from build123d import *

# Parameters (mm, degrees)
SKETCH_1_W          = 15
SKETCH_1_H          = 15
SKETCH_1_W_2        = 12
SKETCH_1_H_2        = 12
EXTRUDE_1_DEPTH     = 135
SKETCH_2_R          = 2.7
CUT_EXTRUDE_1_DEPTH = 25
SKETCH_3_R          = 2.7
SKETCH_3_R_2        = 2.25
CUT_EXTRUDE_2_DEPTH = 25
SKETCH_4_R          = 5
CUT_EXTRUDE_3_DEPTH = 10
SKETCH_5_R          = 5
CUT_EXTRUDE_4_DEPTH = 10
SKETCH_6_R          = 5
CUT_EXTRUDE_5_DEPTH = 10


with BuildPart() as part:
    # ｽｹｯﾁ1 → ﾎﾞｽ - 押し出し1 (new body)
    with BuildSketch(Plane.XY):
        Rectangle(SKETCH_1_W, SKETCH_1_H)
        Rectangle(SKETCH_1_W_2, SKETCH_1_H_2, mode=Mode.SUBTRACT)
    extrude(amount=EXTRUDE_1_DEPTH)

    # ｽｹｯﾁ2 → ｶｯﾄ - 押し出し1 (cut)
    with BuildSketch(Plane(origin=(7.5, 0, 0), x_dir=(0, 0, -1), z_dir=(1, 0, 0))):
        with Locations((-112.5, 0)):
            Circle(SKETCH_2_R)
        with Locations((-22.5, 0)):
            Circle(SKETCH_2_R)
    extrude(amount=-CUT_EXTRUDE_1_DEPTH, mode=Mode.SUBTRACT)

    # ｽｹｯﾁ3 → ｶｯﾄ - 押し出し2 (cut)
    with BuildSketch(Plane(origin=(0, 7.5, 0), x_dir=(1, 0, 0), z_dir=(0, 1, 0))):
        with Locations((0, -7.5)):
            Circle(SKETCH_3_R)
        with Locations((0, -127.5)):
            Circle(SKETCH_3_R_2)
    extrude(amount=-CUT_EXTRUDE_2_DEPTH, mode=Mode.SUBTRACT)

    # ｽｹｯﾁ4 → ｶｯﾄ - 押し出し3 (cut)
    with BuildSketch(Plane(origin=(0, 7.5, 0), x_dir=(1, 0, 0), z_dir=(0, 1, 0))):
        with Locations((0, -7.5)):
            Circle(SKETCH_4_R)
    extrude(amount=-CUT_EXTRUDE_3_DEPTH, mode=Mode.SUBTRACT)

    # ｽｹｯﾁ5 → ｶｯﾄ - 押し出し4 (cut)
    with BuildSketch(Plane(origin=(7.5, 0, 0), x_dir=(0, 0, -1), z_dir=(1, 0, 0))):
        with Locations((-22.5, 0)):
            Circle(SKETCH_5_R)
        with Locations((-112.5, 0)):
            Circle(SKETCH_5_R)
    extrude(amount=-CUT_EXTRUDE_4_DEPTH, mode=Mode.SUBTRACT)

    # ｽｹｯﾁ6 → ｶｯﾄ - 押し出し5 (cut)
    with BuildSketch(Plane(origin=(0, -7.5, 0), x_dir=(-1, 0, 0), z_dir=(0, -1, 0))):
        with Locations((0, -127.5)):
            Circle(SKETCH_6_R)
    extrude(amount=-CUT_EXTRUDE_5_DEPTH, mode=Mode.SUBTRACT)


solid = part.part
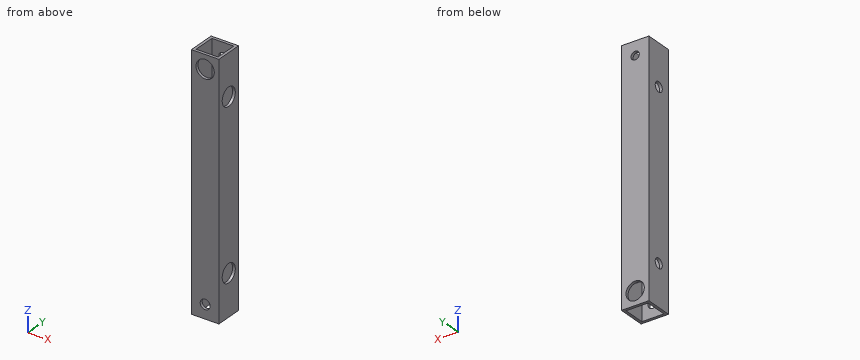
Verification items for the finished model (mm, model axes). Round coordinates to 2 decimals unless told otherwise and drop trailing zeros. Order: outer loops, then holes, each group sorted by start corner. A loop starts at its lowest first (then second) coordinate and runs counter-clockwise, first axis right, second up. Notation, with made-up numbers: (85.5, 10) -> (141.5, 10) arc R15 ccw to (141.5, 32) -> close; hole circle Ø2 at (-1, 70.25). An arc over 180 degrees is marked (long way). Put each result on its own line as item: value.
1) Depth check by flat-ended pin: pin 1 (5 mm diameter, centred on x = 0, z = 127.5, fed in from -Y); pin 2 (8 mm diameter, centred on x = 0, z = 7.5, fed in from -Y). Enter the tip coordinate at first touch or a pass-through.
Final values:
pin 1: stops at y = 6
pin 2: stops at y = -7.5
2) Section check D-D (z = 100). Record the cut outline in (x, y), then the cut area to 3 significant figures.
Final values:
outline: (-7.5, -7.5) -> (7.5, -7.5) -> (7.5, 7.5) -> (-7.5, 7.5) -> close; hole (-6, -6) -> (6, -6) -> (6, 6) -> (-6, 6) -> close
area: 81.0 mm^2
3) Section check A-A (z = 22.5). Record the cut outline in (x, y), then the cut area to 3 significant figures.
Final values:
outline: (-7.5, -7.5) -> (7.5, -7.5) -> (7.5, -5) -> (6, -5) -> (6, -6) -> (-6, -6) -> (-6, -2.7) -> (-7.5, -2.7) -> close; (-7.5, 2.7) -> (-6, 2.7) -> (-6, 6) -> (6, 6) -> (6, 5) -> (7.5, 5) -> (7.5, 7.5) -> (-7.5, 7.5) -> close
area: 57.9 mm^2
4) Material ranges on line 1 (Y direction, x = 6.7, z = 22.5); line 2 (Z direction, x = 0, y = -6.95); line 3 (X direction, y = -3.25, z = 78), recorded low to high.
Final values:
line 1: y = -7.5 to -5, 5 to 7.5
line 2: z = 0 to 4.8, 10.2 to 122.5, 132.5 to 135
line 3: x = -7.5 to -6, 6 to 7.5
5) Section check B-B (y = 0). Record the cut outline in (x, z).
Final values:
outline: (-7.5, 0) -> (-6, 0) -> (-6, 19.8) -> (-7.5, 19.8) -> close; (-7.5, 25.2) -> (-6, 25.2) -> (-6, 109.8) -> (-7.5, 109.8) -> close; (-7.5, 115.2) -> (-6, 115.2) -> (-6, 135) -> (-7.5, 135) -> close; (6, 0) -> (7.5, 0) -> (7.5, 17.5) -> (6, 17.5) -> close; (6, 27.5) -> (7.5, 27.5) -> (7.5, 107.5) -> (6, 107.5) -> close; (6, 117.5) -> (7.5, 117.5) -> (7.5, 135) -> (6, 135) -> close
6) Section check C-C (x = 0). Record the cut outline in (y, z).
Final values:
outline: (-7.5, 0) -> (-6, 0) -> (-6, 4.8) -> (-7.5, 4.8) -> close; (-7.5, 10.2) -> (-6, 10.2) -> (-6, 122.5) -> (-7.5, 122.5) -> close; (-7.5, 132.5) -> (-6, 132.5) -> (-6, 135) -> (-7.5, 135) -> close; (6, 0) -> (7.5, 0) -> (7.5, 2.5) -> (6, 2.5) -> close; (6, 12.5) -> (7.5, 12.5) -> (7.5, 125.25) -> (6, 125.25) -> close; (6, 129.75) -> (7.5, 129.75) -> (7.5, 135) -> (6, 135) -> close
